Design review of the part built by this model. Coordinates are the model's own, in mm. Face numbers are marked on the shaded views. A direction names the side the tool comes from. Coordinates: 2 decimals unless noted, no trailing zeros. Loops run counter-clockwise (first coordinate to the right, second up) from the corner with the lowest first, then second, coordinate; pieces in that order, holes last. Notation, with made-up numbers: (26.5, -14.5) -> (65.5, -14.5) arc R16 cw to (65.5, -0.5) -> close; hole circle Ø8 at (17, 72.25). An arc over 180 degrees is marked (long way). Use CSV: the item, a comma, the result in double quotes.
```python
from build123d import *
from build123d.topology import SkipClean

# Parameters (mm, degrees)
SKETCH1_W           = 110
SKETCH1_H           = 72
SKETCH1_R           = 12.5
SKETCH1_R_2         = 2.25
SKETCH1_R_3         = 8.25
BOSS_EXTRUDE1_DEPTH = 7
BOSS_EXTRUDE2_DEPTH = 15
FILLET2_R           = 10
SKETCH3_R           = 3.75
CUT_EXTRUDE1_DEPTH  = 70.318107302
SKETCH4_W           = 30
SKETCH4_H           = 20
CUT_EXTRUDE2_DEPTH  = 15
CUT_EXTRUDE3_DEPTH  = 68.424031324


with BuildPart() as part:
    # Sketch1 → Boss-Extrude1 (new body)
    with BuildSketch(Plane(origin=(0, 0, 0), x_dir=(1, 0, 0), z_dir=(0, 1, 0))):
        Rectangle(SKETCH1_W, SKETCH1_H)
        with Locations(Location((0, -16.5, 0), (0, 0, 270))):
            Circle(SKETCH1_R, mode=Mode.SUBTRACT)
        with Locations(Location((-15.5, -32, 0), (0, 0, 270))):
            Circle(SKETCH1_R_2, mode=Mode.SUBTRACT)
        with Locations(Location((-15.5, -1, 0), (0, 0, 270))):
            Circle(SKETCH1_R_2, mode=Mode.SUBTRACT)
        with Locations(Location((15.5, -1, 0), (0, 0, 270))):
            Circle(SKETCH1_R_2, mode=Mode.SUBTRACT)
        with Locations(Location((15.5, -32, 0), (0, 0, 270))):
            Circle(SKETCH1_R_2, mode=Mode.SUBTRACT)
        with Locations(Location((25, -16.5, 0), (0, 0, 270))):
            Circle(SKETCH1_R_3, mode=Mode.SUBTRACT)
        with Locations(Location((-5.5, 11.5, 0), (0, 0, 270))):
            Circle(SKETCH1_R_2, mode=Mode.SUBTRACT)
        with Locations(Location((5.5, 11.5, 0), (0, 0, 270))):
            Circle(SKETCH1_R_2, mode=Mode.SUBTRACT)
    extrude(amount=BOSS_EXTRUDE1_DEPTH)

    # Sketch2 → Boss-Extrude2 (add)
    with BuildSketch(Plane(origin=(0, 7, 0), x_dir=(1, 0, 0), z_dir=(0, 1, 0))):
        Polygon((-55, 36), (55, 36), (55, -26), (25, -26), (25, 21), (-25, 21), (-25, -26), (-55, -26), align=None)
    extrude(amount=BOSS_EXTRUDE2_DEPTH)

    # Fillet2
    fillet2_edges = [part.edges().sort_by_distance(p)[0] for p in [
        (-55, 11, -36),
        (55, 11, -36),
    ]]
    fillet(fillet2_edges, radius=FILLET2_R)

    # Sketch3 → Cut-Extrude1 (cut, through all)
    with BuildSketch(Plane.XZ):
        with Locations(Location((40, -26, 0), (0, 0, 270))):
            Circle(SKETCH3_R)
        with Locations(Location((-40, -26, 0), (0, 0, 270))):
            Circle(SKETCH3_R)
        with Locations(Location((-40, 19, 0), (0, 0, 270))):
            Circle(SKETCH3_R)
        with Locations(Location((0, -26, 0), (0, 0, 270))):
            Circle(SKETCH3_R)
        with Locations(Location((40, 19, 0), (0, 0, 270))):
            Circle(SKETCH3_R)
    extrude(amount=-CUT_EXTRUDE1_DEPTH, mode=Mode.SUBTRACT)

    # Sketch4 → Cut-Extrude2 (cut)
    with BuildSketch(Plane(origin=(0, 22, 0), x_dir=(1, 0, 0), z_dir=(0, 1, 0))):
        with Locations((40, 1)):
            Rectangle(SKETCH4_W, SKETCH4_H)
        with Locations((-40, 1)):
            Rectangle(SKETCH4_W, SKETCH4_H)
    extrude(amount=-CUT_EXTRUDE2_DEPTH, mode=Mode.SUBTRACT)

    # Sketch5 → Cut-Extrude3 (cut, through all)
    with SkipClean():  # the faces are left unmerged after this step: merging them gives an invalid solid
        with BuildSketch(Plane.XZ.offset(-7)):
            with BuildLine():
                Line((25, 24.75), (25, 9))
                Line((25, 9), (28.436931771, 9))
                ThreePointArc((28.436931771, 9), (33.060319473, 18.25890591), (25, 24.75))
            make_face()
        extrude(amount=-CUT_EXTRUDE3_DEPTH, mode=Mode.SUBTRACT)


solid = part.part
```
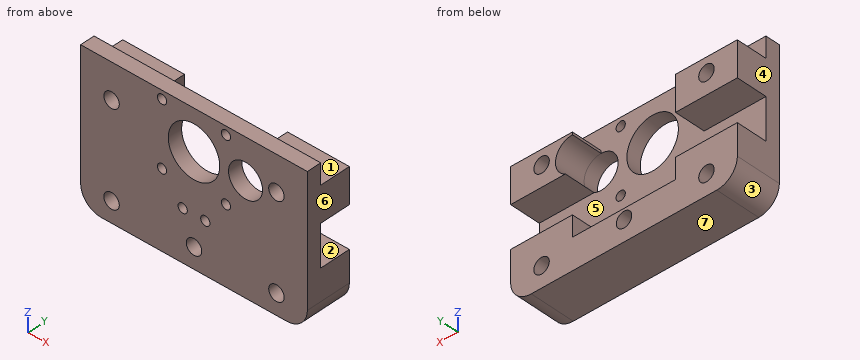
Item 1: Clearance check with flat-ended pins moving along their axes: pin 1 (4.5 mm diameter, centred on x = -40, z = -26, fed in from -Y); pin 2 (10 mm diameter, centred on x = -17, z = 17, fed in from +Y); pin 3 (7.5 mm diameter, centred on x = -40.5, y = 17.5, fed in from +Z). State where each tip first meets the part, or that it passes through.
Checked values:
pin 1,"through"
pin 2,"y = 7"
pin 3,"z = 26"
Item 2: Add section D-D (y = 4.5). State how many separate pieces and enclosed holes the cut face has, then the cut area to 3 significant figures.
Checked values:
separate pieces,"1"
enclosed holes,"13"
area,"6,860 mm^2"
Item 3: Machinability: for the marked faces 1, 2 and 3, which of the approach directions +Z, -Z, +X, -X, +Y, -Y give a long, thin tool a straight path to every point of the face, cutting with its end or side? Answer none if there is none.
Checked values:
face 1,"+Z, +X, -X, +Y"
face 2,"+X, -X, +Y"
face 3,"-Z, -X, +Y, -Y"
Item 4: Add section C-C (x = 0). Give the boundary of the cut face in (y, z), then the cut area to 3 significant figures.
Checked values:
outline,"(0, -36) -> (22, -36) -> (22, -29.75) -> (0, -29.75) -> close; (0, -22.25) -> (22, -22.25) -> (22, -21) -> (7, -21) -> (7, 4) -> (0, 4) -> close; (0, 29) -> (7, 29) -> (7, 36) -> (0, 36) -> close"
area,"389 mm^2"
Item 5: Add section A-A (y = 18.5). Give the boundary of the cut face in (x, z), then the cut area to 3 significant figures.
Checked values:
outline,"(-55, -26) arc R10 ccw to (-45, -36) -> (45, -36) arc R10 ccw to (55, -26) -> (55, -11) -> (25, -11) -> (25, -21) -> (-25, -21) -> (-25, -11) -> (-55, -11) -> close; (-55, 9) -> (-25, 9) -> (-25, 26) -> (-55, 26) -> close; (25, 24.75) arc R8.25 cw to (28.44, 9) -> (55, 9) -> (55, 26) -> (25, 26) -> close; hole circle Ø7.5 at (-40, -26); hole circle Ø7.5 at (-40, 19); hole circle Ø7.5 at (0, -26); hole circle Ø7.5 at (40, -26); hole circle Ø7.5 at (40, 19)"
area,"2,900 mm^2"
Item 6: Draft analysis for pull direction X (two halves, no side actions). For the marked faces 4, 5, 6 and 7, state which applies: pulls with the +X half, pulls with the -X half, needs draft (parallel to the pull), parting line crosses it, or undercut.
Checked values:
face 4,"pulls with the -X half"
face 5,"undercut"
face 6,"pulls with the +X half"
face 7,"needs draft"
Item 7: To check wall thickness, follow line 1 along X through (y, z) = (10.25, -26); line 2 along X through (y, z) = (5.5, -11.5); line 3 along Z through (x, y) = (44.5, 13.5). State the ranges of each line that lie inside material, in increasing order.
Checked values:
line 1,"-55 to -43.75, -36.25 to -3.75, 3.75 to 36.25, 43.75 to 55"
line 2,"-55 to -7.75, -3.25 to 3.25, 7.75 to 55"
line 3,"-36 to -11, 9 to 26"
Item 8: Add section B-B (z = 1). Give the boundary of the cut face in (x, y), then the cut area to 3 significant figures.
Checked values:
outline,"(-55, 0) -> (-17.75, 0) -> (-17.75, 7) -> (-55, 7) -> close; (-13.25, 0) -> (13.25, 0) -> (13.25, 7) -> (-13.25, 7) -> close; (17.75, 0) -> (55, 0) -> (55, 7) -> (17.75, 7) -> close"
area,"707 mm^2"
